Autodesk Fusion 360 part; units mm, degrees
sketch "Sketch1" plane through (0, 0, 0) normal (0, 1, 0) x (1, 0, 0)
  line L0 (0, -25) -> (23, -25)
  line L1 (25, -23) -> (25, 23)
  line L2 (23, 25) -> (0, 25)
  line L3 (0, -25) -> (-23, -25)
  line L4 (-25, -23) -> (-25, 23)
  line L5 (-23, 25) -> (0, 25)
  line L6 (0, -23) -> (-23, -23)
  line L7 (-23, -23) -> (-23, 23)
  line L8 (-23, 23) -> (0, 23)
  line L9 (23, 23) -> (0, 23)
  line L10 (23, -23) -> (23, 23)
  line L11 (0, -23) -> (23, -23)
  arc A0 (23, -25) -> (25, -23) centre (23, -23) ccw
  arc A1 (-25, -23) -> (-23, -25) centre (-23, -23) ccw
  arc A2 (-23, 25) -> (-25, 23) centre (-23, 23) ccw
  arc A3 (25, 23) -> (23, 25) centre (23, 23) ccw
  line L12 (73, 23) -> (50, 23)
  line L13 (73, 25) -> (50, 25)
  line L14 (50, -23) -> (73, -23)
  line L15 (50, -23) -> (27, -23)
  line L16 (50, -25) -> (73, -25)
  arc A4 (25, -23) -> (27, -25) centre (27, -23) ccw
  line L17 (27, 25) -> (50, 25)
  arc A5 (75, 23) -> (73, 25) centre (73, 23) ccw
  line L18 (73, -23) -> (73, 23)
  line L19 (25, -23) -> (25, 23)
  line L20 (27, -23) -> (27, 23)
  arc A6 (73, -25) -> (75, -23) centre (73, -23) ccw
  arc A7 (27, 25) -> (25, 23) centre (27, 23) ccw
  line L21 (50, -25) -> (27, -25)
  line L22 (75, -23) -> (75, 23)
  line L23 (27, 23) -> (50, 23)
  point P0 (25, -25)
  point P1 (25, 25)
  point P2 (75, -25)
  point P3 (75, 25)
  point P4 (50, 0)
  dimension "d1" = 25
  dimension "d2" = 25
  dimension "d3" = 50
  dimension "d4" = 2
  dimension "d7" = 2
  dimension "d8" = 2
  dimension "d9" = 2
  dimension "d10" = 2
  dimension "d11" = 2
  dimension "d12" = 25
  dimension "d13" = 25
  dimension "d14" = 50
  dimension "d15" = 2
  dimension "d16" = 2
  dimension "d17" = 2
  dimension "d18" = 2
extrude "Extrude2" add sketch "Sketch1" along normal blind 200
sketch "Sketch2" plane through (0, 0, 25) normal (0, 0, 1) x (-1, 0, 0)
  line L0 (23, 0) -> (-23, 0)
  line L1 (-23, 0) -> (-23, -200)
  line L2 (-23, -200) -> (23, -200)
  line L3 (23, -200) -> (23, 0)
  line L4 (25, 0) -> (-75, 0)
  line L5 (-75, 0) -> (-75, -200)
  line L6 (-75, -200) -> (25, -200)
  line L7 (25, -200) -> (25, 0)
  dimension "d21" = 100
  dimension "d22" = 200
extrude "Extrude3" add sketch "Sketch2" along normal blind 5 contours L0 L1 L2 L3 L4 L6 | L1 L4 L5 L6
sketch "Sketch3" plane through (0, 0, 30) normal (0, 0, 1) x (-1, 0, 0)
  line L0 (-75, -200) -> (23, -200)
  line L1 (23, -200) -> (23, 0)
  line L2 (23, 0) -> (-75, 0)
  line L3 (-75, 0) -> (-75, -200)
  line L4 (-75, 0) -> (-65, 0)
  line L5 (-65, 0) -> (-65, -10)
  line L6 (-65, -10) -> (-75, -10)
  line L7 (-75, -10) -> (-75, 0)
  circle A0 centre (-65, -10) radius 3
  circle A1 centre (-30, -10) radius 3
  circle A2 centre (5, -10) radius 3
  circle A3 centre (-65, -55) radius 3
  circle A4 centre (-65, -100) radius 3
  circle A5 centre (-65, -145) radius 3
  circle A6 centre (-65, -190) radius 3
  circle A7 centre (-30, -190) radius 3
  circle A8 centre (5, -190) radius 3
  dimension "d25" = 10
  dimension "d26" = 10
  dimension "d27" = 6
  dimension "d30" = 70
  dimension "d31" = -180
extrude "Extrude4" cut sketch "Sketch3" against normal blind 7 contours L5 L6 A0 | L5 L6 A0 | A1 | A2 | A3 | A4 | A5 | A6 | A7 | A8
chamfer "Chamfer1" distance 0.5 angle 45 1 edges at (-2.203, 188.9152, 30)
chamfer "Chamfer2" distance 0.5 angle 45 1 edges at (32.797, 188.9152, 30)
chamfer "Chamfer3" distance 0.5 angle 45 1 edges at (67.797, 188.9152, 30)
chamfer "Chamfer4" distance 0.5 angle 45 1 edges at (67.797, 143.9152, 30)
chamfer "Chamfer5" distance 0.5 angle 45 1 edges at (67.797, 98.9152, 30)
chamfer "Chamfer6" distance 0.5 angle 45 1 edges at (67.797, 53.9152, 30)
chamfer "Chamfer7" distance 0.5 angle 45 1 edges at (67.797, 8.9152, 30)
chamfer "Chamfer8" distance 0.5 angle 45 1 edges at (32.797, 8.9152, 30)
chamfer "Chamfer9" distance 0.5 angle 45 1 edges at (-2.203, 8.9152, 30)
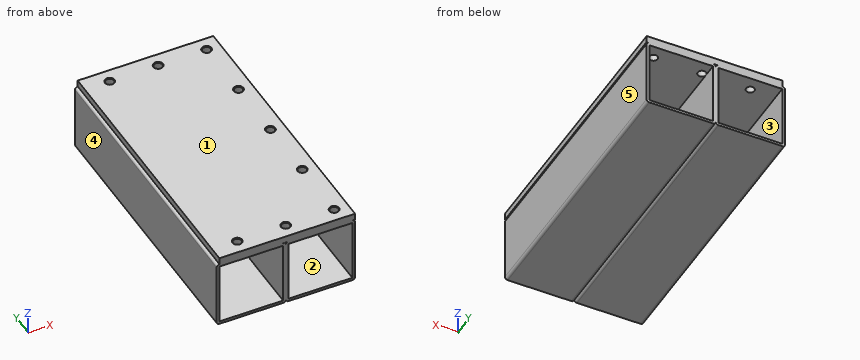
Input: part model. Units: mm. Frame: model coordinates. Face numbers are marked on the shaded views. A direction names the side the tool comes from. Round coordinates to 2 decimals unless told otherwise and drop trailing zeros. Loops run counter-clockwise (first coordinate to the right, second up) from the corner with the lowest first, then second, coordinate; pieces in that order, holes last. Notation, with made-up numbers: M 21.25,54.25 L 68.25,54.25 A22 ccw 68.25,61.25 Z; hole C 28,-26.5 d3. An arc over 180 degrees is marked long. Answer in a Markdown table with one row per item. Add a question column.
1. Section B-B (z = -13). Output: boundary loops of the cut face in (x, y).
2. Ray query, probe 1 along Y at (x, z) = (65, 28.25); probe 2 along X at (y, z) = (142, -7.5); probe 3 along Y at (x, z) = (-5, 27). Return the intervals inside material, ascending.
3. Mould query, pull axis X, two halves, no side actions, for the marked faces 3, 4 and 5. Classes: released by +X, released by -X, zero draft, split by the parting line, or undercut.
4. Section C-C (y = 145). Give the number of separate pieces and of enclosed holes in the cut face, and give its area (3 significant figures).
5. Section A-A (x = 30). Output: boundary loops of the cut face in (y, z).
6. Contact query for flat-ended pins moving along their axis: pin 1 (1.2 mm diameter, centred on x = 26, y = 50.5, fed in from -Z); pin 2 (1 mm diameter, centred on x = 74.5, y = 146, fed in from -Z); pin 3 (12 mm diameter, centred on x = 50.5, z = 16, fed in from +Y); pin 4 (5.5 mm diameter, centred on y = 96, z = 27.5, fed in from -X). Output: stop coordinate, or through.
7. Section D-D (x = 51). Output: boundary loops of the cut face in (y, z), and give its area (3 significant figures).
8. Set-up query: the marked faces 1 and 2. Return all of +Z, -Z, +X, -X, +Y, -Y with unobstructed straight access to the full face (end or side cutting, diameter ignored); none if empty.
Values follow:
| question | item | result |
|---|---|---|
| 1 | outline | M -25,0 L -23,0 L -23,200 L -25,200 Z; M 23,0 L 27,0 L 27,200 L 23,200 Z; M 73,0 L 75,0 L 75,200 L 73,200 Z |
| 2 | probe 1 | 0 to 7, 13 to 52, 58 to 97, 103 to 142, 148 to 187, 193 to 200 |
| 2 | probe 2 | -25 to -23, 23 to 27, 73 to 75 |
| 2 | probe 3 | 0 to 7, 13 to 187, 193 to 200 |
| 3 | face 3 | undercut |
| 3 | face 4 | released by -X |
| 3 | face 5 | released by +X |
| 4 | separate pieces | 1 |
| 4 | enclosed holes | 2 |
| 4 | area | 1,210 mm^2 |
| 5 | outline | M 0,-25 L 200,-25 L 200,-23 L 0,-23 Z; M 0,23 L 7,23 L 7,29.5 L 6.5,30 L 0,30 Z; M 13,23 L 187,23 L 187,29.5 L 186.5,30 L 13.5,30 L 13,29.5 Z; M 193,23 L 200,23 L 200,30 L 193.5,30 L 193,29.5 Z |
| 6 | pin 1 | z = -24.96 |
| 6 | pin 2 | z = -24.73 |
| 6 | pin 3 | through |
| 6 | pin 4 | x = -23.97 |
| 7 | outline | M 0,-25 L 200,-25 L 200,-23 L 0,-23 Z; M 0,23 L 200,23 L 200,30 L 0,30 Z |
| 7 | area | 1,800 mm^2 |
| 8 | face 1 | +Z, +X, -X, +Y, -Y |
| 8 | face 2 | +Y, -Y |
